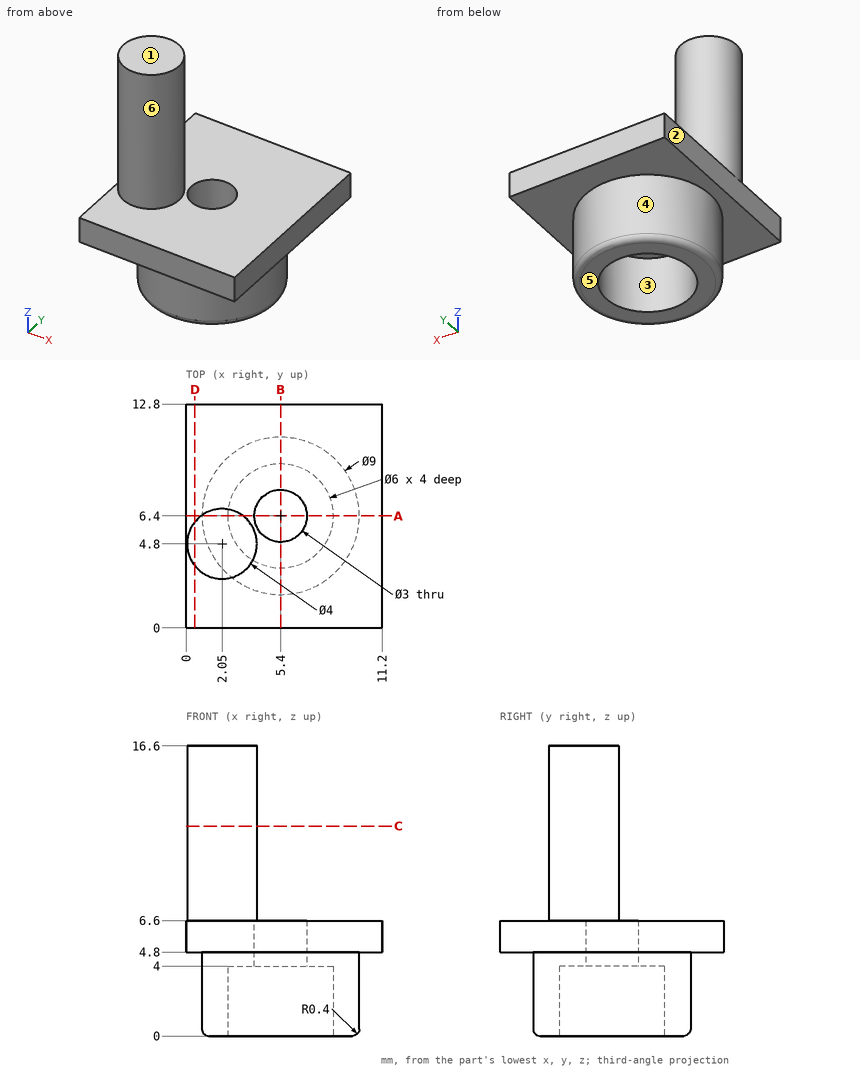
Part print with two shaded views. Sizes in mm from the minimum x, y, z corner. A direction names the side the tool comes from. Coordinates: 2 decimals unless noted, no trailing zeros. Order: outer loops, then holes, each group sorted by start corner. A loop starts at its lowest first (then second) coordinate and runs counter-clockwise, first axis right, second up.
(1) Drill centre lines: L1, parallel to Y at x = 5.4, z = 4.9; L2, parallel to Y at x = 5.4, z = 1.55; L3, parallel to Z at x = 6, y = 4.25. Where is each one in solid material? Low to high.
Solution:
L1: y = 0 to 4.9, 7.9 to 12.8
L2: y = 1.9 to 3.4, 9.4 to 10.9
L3: z = 4 to 6.6
(2) Which spindle directions (+Z, -Z, +X, -X, +Y, -Y) get a long thin tool onto all of the face, cutting with end or side? Do the marked faces 4, 5 and 6. Say none if no direction does.
Solution:
face 4: -Z
face 5: -Z, +X, -X, +Y, -Y
face 6: +Z
(3) Mould opens along X. For the marked faces 1, 2 and 3 say: released by +X, released by -X, zero draft, split by the parting line, or undercut.
Solution:
face 1: zero draft
face 2: released by -X
face 3: undercut
(4) Pin check, flat tips, straight feed: pin 1 Ø1 at (y, z) = (6.5, 10.5) entering from -X; pin 2 Ø6 at (y, z) = (11, 10.5) entering from +X; pin 3 Ø3 at (x, y) = (5, 6) entering from -Z; pin 4 Ø4 at (y, z) = (6, 12) entering from +X. Stop position of each tip, or through.
Solution:
pin 1: stops at x = 0.45
pin 2: passes through
pin 3: stops at z = 4
pin 4: stops at x = 4.05
(5) Saw through at A-A, the plane y = 6.4. Write the cut outline in (x, z).
Solution:
outline: (0, 4.8) - (0.9, 4.8) - (0.9, 0.4) arc R0.4 ccw to (1.3, 0) - (2.4, 0) - (2.4, 4) - (3.9, 4) - (3.9, 6.6) - (3.25, 6.6) - (3.25, 16.6) - (0.85, 16.6) - (0.85, 6.6) - (0, 6.6) - close; (6.9, 4) - (8.4, 4) - (8.4, 0) - (9.5, 0) arc R0.4 ccw to (9.9, 0.4) - (9.9, 4.8) - (11.2, 4.8) - (11.2, 6.6) - (6.9, 6.6) - close
(6) Saw through at D-D, the plane x = 0.5. Write the cut outline in (y, z), and give its area (3 significant figures).
Solution:
outline: (0, 4.8) - (12.8, 4.8) - (12.8, 6.6) - (6.06, 6.6) - (6.06, 16.6) - (3.54, 16.6) - (3.54, 6.6) - (0, 6.6) - close
area: 48.3 mm2
(7) Saw through at B-B, the plane x = 5.4. Write the cut outline in (y, z).
Solution:
outline: (0, 4.8) - (1.9, 4.8) - (1.9, 0.4) arc R0.4 ccw to (2.3, 0) - (3.4, 0) - (3.4, 4) - (4.9, 4) - (4.9, 6.6) - (0, 6.6) - close; (7.9, 4) - (9.4, 4) - (9.4, 0) - (10.5, 0) arc R0.4 ccw to (10.9, 0.4) - (10.9, 4.8) - (12.8, 4.8) - (12.8, 6.6) - (7.9, 6.6) - close
(8) Saw through at C-C, the plane z = 12. Write the cut outline in (x, y), and give its area (3 significant figures).
Solution:
outline: circle Ø4 at (2.05, 4.8)
area: 12.6 mm2
